Work out the finished part from the listing and answer in its coordinate system (mm). A direction names the side the tool comes from. Give positions to 0.01 mm unless a question says otherwise; leave off trailing zeros. Loops run counter-clockwise (first coordinate to the right, second up) from the corner with the lowest first, then second, coordinate; pieces in that order, holes last. Notation, with made-up numbers: (66.5, 77.5) - (79.5, 77.5) arc R21 cw to (79.5, 81.5) - close; hole circle Ø11 at (50, -25). An arc over 180 degrees is marked (long way). One line per item, written item: value.
from build123d import *

# Parameters (mm, degrees)
BOSS_EXTRUDE1_DEPTH = 25.4
FILLET1_R           = 12.7
SKETCH2_R           = 3.175
CUT_EXTRUDE1_DEPTH  = 18.17675
SKETCH3_R           = 2.4892
CUT_EXTRUDE2_DEPTH  = 3.54


with BuildPart() as part:
    # Sketch1 → Boss-Extrude1 (new body)
    with BuildSketch(Plane.XY):
        Polygon((-10.16, -12.7), (-10.16, 12.7), (-27.33675, 12.7), (-27.33675, 10.16), (-12.7, 10.16), (-12.7, -12.7), align=None)
    extrude(amount=BOSS_EXTRUDE1_DEPTH)

    # Fillet1
    fillet1_edges = [part.edges().sort_by_distance(p)[0] for p in [
        (-11.43, -12.7, 0),
    ]]
    fillet(fillet1_edges, radius=FILLET1_R)

    # Sketch2 → Cut-Extrude1 (cut, through all)
    with BuildSketch(Plane(origin=(-10.16, 0, 0), x_dir=(0, 0, -1), z_dir=(1, 0, 0))):
        with Locations((-10.45493597, -2.24506403)):
            Circle(SKETCH2_R)
    extrude(amount=-CUT_EXTRUDE1_DEPTH, mode=Mode.SUBTRACT)

    # Sketch3 → Cut-Extrude2 (cut, through all)
    with BuildSketch(Plane(origin=(-0.012018133, 10.16, 0), x_dir=(1, 0, 0), z_dir=(0, -1, 0))):
        with Locations((-19.672981867, 19.05)):
            Circle(SKETCH3_R)
        with Locations((-19.672981867, 6.35)):
            Circle(SKETCH3_R)
    extrude(amount=-CUT_EXTRUDE2_DEPTH, mode=Mode.SUBTRACT)


solid = part.part
1. The mould has two halves that part along Z. Classify faces 1 (the cylindrical face through (-20.22, 11.41, 16.62)), 2 (the flat face through (-27.337, 11, 13)), 3 (the flat face through (-16, 12, 0)): released by +Z, released by -Z, zero draft, split by the parting line, or undercut.
Output:
face 1: undercut
face 2: zero draft
face 3: released by -Z
2. Flat-ended cylindrical pins translate along their axes: pin 1 Ø5 at (y, z) = (6, 22.5) entering from -X; pin 2 Ø7.5 at (x, z) = (-21, 14.5) entering from -Y; pin 3 Ø5 at (y, z) = (-2.25, 10.45) entering from +X. Find the tip coordinate at first contact, or state that the pin passes through.
Output:
pin 1: stops at x = -12.7
pin 2: stops at y = 10.16
pin 3: passes through
3. For faces 4 (the flat face through (-20, 10.16, 13)), 5 (the flat face through (-19, 12.7, 13)), determine the directions among +Z, -Z, +X, -X, +Y, -Y from which every point of the face is accessible in a straight line to the end or side of a thin tool.
Output:
face 4: +Z, -Z, -X, -Y
face 5: +Z, -Z, +X, -X, +Y
4. Section D-D (z = 7.75) is taken. Write down the section's boundary in (x, y).
Output:
outline: (-27.34, 10.16) - (-21.74, 10.16) - (-21.74, 12.7) - (-27.34, 12.7) - close; (-17.63, 10.16) - (-12.7, 10.16) - (-12.7, -0.58) - (-10.16, -0.58) - (-10.16, 12.7) - (-17.63, 12.7) - close; (-12.7, -11.7) - (-10.16, -11.7) - (-10.16, -3.91) - (-12.7, -3.91) - close
5. Section A-A (z = 19.05) is taken. Write down the section's boundary in (x, y), and give its area (3 significant figures).
Output:
outline: (-27.34, 10.16) - (-22.17, 10.16) - (-22.17, 12.7) - (-27.34, 12.7) - close; (-17.2, 10.16) - (-12.7, 10.16) - (-12.7, -12.7) - (-10.16, -12.7) - (-10.16, 12.7) - (-17.2, 12.7) - close
area: 89.0 mm²
6. Find the intervals of material crossed by line 1 along Y through (x, z) = (-19.5, 12); line 2 along X through (y, z) = (3.5, 19.75), in increasing order.
Output:
line 1: y = 10.16 to 12.7
line 2: x = -12.7 to -10.16
7. Section C-C (y = -3.25) is taken. Write down the section's boundary in (x, z), and give its area (3 significant figures).
Output:
outline: (-12.7, 0.42) - (-10.16, 0.42) - (-10.16, 7.44) - (-12.7, 7.44) - close; (-12.7, 13.47) - (-10.16, 13.47) - (-10.16, 25.4) - (-12.7, 25.4) - close
area: 48.1 mm²
8. Section B-B (x = -18) is taken. Write down the section's boundary in (y, z), and give its area (3 significant figures).
Output:
outline: (10.16, 0) - (12.7, 0) - (12.7, 4.52) - (10.16, 4.52) - close; (10.16, 8.18) - (12.7, 8.18) - (12.7, 17.22) - (10.16, 17.22) - close; (10.16, 20.88) - (12.7, 20.88) - (12.7, 25.4) - (10.16, 25.4) - close
area: 45.9 mm²
